Work out the finished part from the listing and answer in its coordinate system (mm). Round coordinates to 2 decimals unless told otherwise and drop trailing zeros. Order: outer loops, then holes, each group sorted by start corner. A loop starts at its lowest first (then second) coordinate and runs counter-clockwise, first axis right, second up. Notation, with made-up numbers: M -26.5,-16.75 L -17.5,-16.75 A36 ccw -17.5,17.25 Z; hole C -31.75,-17 d7. An arc over 180 degrees is marked long. Return JSON: item names as keys, results as strings.
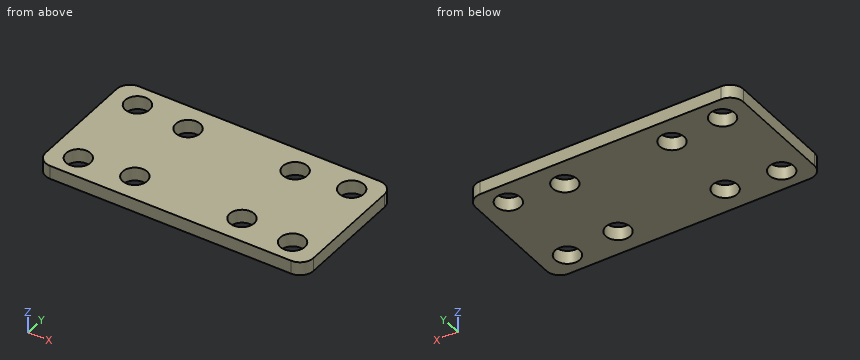
Autodesk Inventor part; units mm, degrees
ref_plane "YZ Plane" through (0, 0, 0) normal (1, 0, 0) x (0, 1, 0)
ref_plane "XZ Plane" through (0, 0, 0) normal (0, 1, 0) x (-1, 0, 0)
ref_plane "XY Plane" through (0, 0, 0) normal (0, 0, 1) x (1, 0, 0)
sketch "Sketch1" plane through (0, 0, 0) normal (0, 0, 1) x (1, 0, 0)
  line L0 (-30, -15) -> (30, -15)
  line L1 (30, -15) -> (30, 15)
  line L2 (30, 15) -> (-30, 15)
  line L3 (-30, 15) -> (-30, -15)
  line L4 (-30, -15) -> (30, 15) construction
  line L5 (30, -15) -> (-30, 15) construction
  line L6 (-12, -9) -> (12, -9)
  line L7 (12, -9) -> (12, 9)
  line L8 (12, 9) -> (-12, 9)
  line L9 (-12, 9) -> (-12, -9)
  line L10 (-12, -9) -> (12, 9) construction
  line L11 (12, -9) -> (-12, 9) construction
  circle A0 centre (-12, 9) radius 2.75
  circle A1 centre (12, 9) radius 2.75
  circle A2 centre (-12, -9) radius 2.75
  circle A3 centre (12, -9) radius 2.75
  point P0 (0, 0)
  dimension "d0" = 60
  dimension "d1" = 30
  dimension "d2" = 24
  dimension "d3" = 18
  dimension "d4" = 5.5
  dimension "d5" = 5.5
  dimension "d6" = 5.5
  dimension "d7" = 5.5
extrude "Extrusion1" add sketch "Sketch1" along normal blind 3 contours L3 L2 L1 L0 | A2 L9 A0 L8 A1 L7 A3 L6
sketch "Sketch2" plane through (0, 0, 3) normal (0, 0, 1) x (1, 0, 0)
  circle A0 centre (-24, 10) radius 2.75
  circle A1 centre (-24, -10) radius 2.75
  line L0 (-30, 15) -> (-30, -15)
  circle A2 centre (24, 10) radius 2.75
  circle A3 centre (24, -10) radius 2.75
  line L1 (30, -15) -> (30, 15)
  point P0 (0, 0)
  dimension "d10" = 5.5
  dimension "d11" = 5.5
  dimension "d12" = 10
  dimension "d13" = 6
  dimension "d14" = 6
  dimension "d15" = 10
  dimension "d16" = 5.5
  dimension "d17" = 5.5
  dimension "d18" = 20
  dimension "d19" = 10
  dimension "d20" = 6
  dimension "d21" = 6
extrude "Extrusion2" cut sketch "Sketch2" against normal blind 3
fillet "Fillet1" radius 3 4 edges at (30, 15, 1.5) (30, -15, 1.5) (-30, -15, 1.5) (-30, 15, 1.5)
properties part number "De lot vitme"
Item 1: Find section B-B (z = 2.4). State how many separate pieces and enclosed holes the cut face has, plus the area to 3 significant figures.
Output:
{"separate pieces": "1", "enclosed holes": "8", "area": "1,600 mm^2"}
Item 2: Consider line 1 along Y through (x, z) = (-24, 0.9); line 2 along X through (y, z) = (-10.5, 2.1); line 3 along Y through (x, z) = (-13, 1.65). Determine where each line is inside the solid, lowest interval first. Write a range as [from, to].
Output:
{"line 1": "y = [-15, -12.75], [-7.25, 7.25], [12.75, 15]", "line 2": "x = [-30, -26.7], [-21.3, -14.3], [-9.7, 9.7], [14.3, 21.3], [26.7, 30]", "line 3": "y = [-15, -11.56], [-6.44, 6.44], [11.56, 15]"}
Item 3: Find section A-A (x = 12). Determine the outline of the cut face in (y, z).
Output:
{"outline": "M -15,0 L -11.75,0 L -11.75,3 L -15,3 Z; M -6.25,0 L 6.25,0 L 6.25,3 L -6.25,3 Z; M 11.75,0 L 15,0 L 15,3 L 11.75,3 Z"}
Item 4: This flat-tipped pin is pushed along its axis until it touches: pin 1 (9 mm diameter, centred on x = 24, y = 10, fed in from -Z). Where does it stop, or does it pass through?
Output:
{"pin 1": "stops at z = 0"}
Item 5: Find section C-C (y = -10). Determine the outline of the cut face in (x, z), plus the area to 3 significant figures.
Output:
{"outline": "M -30,0 L -26.75,0 L -26.75,3 L -30,3 Z; M -21.25,0 L -14.56,0 L -14.56,3 L -21.25,3 Z; M -9.44,0 L 9.44,0 L 9.44,3 L -9.44,3 Z; M 14.56,0 L 21.25,0 L 21.25,3 L 14.56,3 Z; M 26.75,0 L 30,0 L 30,3 L 26.75,3 Z", "area": "116 mm^2"}
